Geometry check sheet. Reference: the model listing, model coordinates, mm. A direction names the side the tool comes from. Round coordinates to 2 decimals unless told otherwise and drop trailing zeros. Order: outer loops, then holes, each group sorted by start corner. A loop starts at its lowest first (then second) coordinate and runs counter-clockwise, first axis right, second up.
(1) Gauge pin test, flat ends, axial feed: P1, Ø1.6, axis at x = 0, z = -6.5, coming from the -Y side (3 decimals); P2, Ø2, axis at y = 1.5, z = -11.5, coming from the -X side. Record the tip position at first contact, or that the pin passes through.
(2) Cross-section at B-B on z = 0. Enter the section's corners in (x, y), and give its area (3 significant figures).
(3) Draft check along Z on faces 1 (the face through (0, 0, -20.002)), 2 (the face through (0, -3.175, -15)), 3 (the face through (0, 0, 4.762)), 4 (the face through (0, 6.35, -8)). Enter one of: pulls with the +Z half, pulls with the -Z half, needs draft (parallel to the pull), parting line crosses it, or undercut.
(4) Cross-section at A-A on y = 0. Enter the section's corners in (x, z) (1 decimal), and give its area (3 significant figures).
(5) Cross-section at C-C on y = -2. Enter the section's corners in (x, z) (1 decimal).
(6) Thickness scan on L1, parallel to Z at x = -0.7, y = -2 (1 decimal); L2, parallel to Z at x = 1.05, y = 2.75; L3, parallel to Y at x = 0.65, z = -8.75 (3 decimals). Record the ranges inside material, lowest first.
(7) Set-up check for faces 5 (the face through (0, 0.508, -14)), 6 (the face through (0, -6.35, 0)), 7 (the face through (0, -3.175, -7)): record each of +Z, -Z, +X, -X, +Y, -Y from which the full face is reachable in a straight line by a thin tool's end or side.
from build123d import *

# Parameters (mm, degrees)
SKETCH2_R                = 1.5875
BOSS_EXTRUDE1_DEPTH      = 1.5875
BOSS_EXTRUDE1_DEPTH_BACK = 1.5875


with BuildPart() as part:
    # Sketch2 → Boss-Extrude1 (new body, two sides)
    with BuildSketch(Plane(origin=(0, 0, 0), x_dir=(0, 0, -1), z_dir=(1, 0, 0))) as boss_extrude1_sk:
        Polygon((-4.7625, 6.35), (-4.7625, -6.35), (4.7625, -6.35), (4.7625, -3.175), (9.525, -3.175), (9.525, 0.508), (7.874, 0.508), (7.874, 3.302), (14.351, 3.302), (14.351, 0.508), (12.7, 0.508), (12.7, -3.175), (16.8275, -3.175), (16.8275, -6.35), (20.0025, -6.35), (20.0025, 6.35), align=None)
        Circle(SKETCH2_R, mode=Mode.SUBTRACT)
    extrude(amount=BOSS_EXTRUDE1_DEPTH)
    extrude(boss_extrude1_sk.sketch, amount=-BOSS_EXTRUDE1_DEPTH_BACK)


solid = part.part
Found:
1. P1: stops at y = -3.175
1. P2: passes through
2. outline: (-1.59, -6.35) - (1.59, -6.35) - (1.59, -1.59) - (-1.59, -1.59) - close; (-1.59, 1.59) - (1.59, 1.59) - (1.59, 6.35) - (-1.59, 6.35) - close
2. area: 30.2 mm2
3. face 1: pulls with the -Z half
3. face 2: undercut
3. face 3: pulls with the +Z half
3. face 4: needs draft
4. outline: (-1.6, -20) - (1.6, -20) - (1.6, -12.7) - (-1.6, -12.7) - close; (-1.6, -9.5) - (1.6, -9.5) - (1.6, -1.6) - (-1.6, -1.6) - close; (-1.6, 1.6) - (1.6, 1.6) - (1.6, 4.8) - (-1.6, 4.8) - close
4. area: 58.5 mm2
5. outline: (-1.6, -20) - (1.6, -20) - (1.6, -12.7) - (-1.6, -12.7) - close; (-1.6, -9.5) - (1.6, -9.5) - (1.6, 4.8) - (-1.6, 4.8) - close
6. L1: z = -20 to -12.7, -9.5 to 4.8
6. L2: z = -20 to -14.35, -7.87 to 4.76
6. L3: y = -3.175 to 0.508, 3.302 to 6.35
7. face 5: +X, -X
7. face 6: +Z, -Z, +X, -X, -Y
7. face 7: +X, -X, -Y
